```python
from build123d import *

# Parameters (mm, degrees)
SKETCH1_W           = 20
SKETCH1_H           = 50
BOSS_EXTRUDE1_DEPTH = 70
SKETCH2_R           = 2
SKETCH2_R_2         = 11.5
CUT_EXTRUDE2_DEPTH  = 60
SKETCH4_W           = 37
SKETCH4_H           = 15
CUT_EXTRUDE3_DEPTH  = 60
SKETCH8_R           = 2
CUT_EXTRUDE5_DEPTH  = 15
SKETCH9_W           = 42
SKETCH9_H           = 42
CUT_EXTRUDE6_DEPTH  = 6
CUT_EXTRUDE8_DEPTH  = 30
SKETCH12_W          = 20
SKETCH12_H          = 5
BOSS_EXTRUDE2_DEPTH = 10
BOSS_EXTRUDE3_DEPTH = 20
SKETCH15_R          = 2
CUT_EXTRUDE9_DEPTH  = 10
SKETCH17_R          = 3.5
CUT_EXTRUDE11_DEPTH = 8
SKETCH18_R          = 3.5
CUT_EXTRUDE12_DEPTH = 50


with BuildPart() as part:
    # Sketch1 → Boss-Extrude1 (new body)
    with BuildSketch(Plane(origin=(0, 0, 0), x_dir=(1, 0, 0), z_dir=(0, 1, 0))):
        with Locations((-10, -25)):
            Rectangle(SKETCH1_W, SKETCH1_H)
    extrude(amount=BOSS_EXTRUDE1_DEPTH)

    # Sketch2 → Cut-Extrude2 (cut)
    with BuildSketch(Plane(origin=(0, 0, 0), x_dir=(0, 0, -1), z_dir=(1, 0, 0))):
        with Locations((-9.5, 58)):
            Circle(SKETCH2_R)
        with Locations((-25, 42.5)):
            Circle(SKETCH2_R_2)
        with Locations((-9.5, 27)):
            Circle(SKETCH2_R)
        with Locations((-40.5, 27)):
            Circle(SKETCH2_R)
        with Locations((-40.5, 58)):
            Circle(SKETCH2_R)
    extrude(amount=-CUT_EXTRUDE2_DEPTH, mode=Mode.SUBTRACT)

    # Sketch4 → Cut-Extrude3 (cut)
    with BuildSketch(Plane(origin=(0, 0, 0), x_dir=(0, 0, -1), z_dir=(1, 0, 0))):
        with Locations((-31.5, 7.5)):
            Rectangle(SKETCH4_W, SKETCH4_H)
    extrude(amount=-CUT_EXTRUDE3_DEPTH, mode=Mode.SUBTRACT)

    # Sketch8 → Cut-Extrude5 (cut)
    with BuildSketch(Plane(origin=(0, 0, 0), x_dir=(-1, 0, 0), z_dir=(0, 0, -1))):
        with Locations((15, 6)):
            Circle(SKETCH8_R)
        with Locations((5, 6)):
            Circle(SKETCH8_R)
    extrude(amount=-CUT_EXTRUDE5_DEPTH, mode=Mode.SUBTRACT)

    # Sketch9 → Cut-Extrude6 (cut)
    with BuildSketch(Plane(origin=(0, 0, 0), x_dir=(0, 0, -1), z_dir=(1, 0, 0))):
        with Locations((-25, 42.5)):
            Rectangle(SKETCH9_W, SKETCH9_H)
    extrude(amount=-CUT_EXTRUDE6_DEPTH, mode=Mode.SUBTRACT)

    # Sketch11 → Cut-Extrude8 (cut)
    with BuildSketch(Plane(origin=(0, 0, 0), x_dir=(0, 0, -1), z_dir=(1, 0, 0))):
        Polygon((-7, 0), (0, 0), (0, 15), align=None)
    extrude(amount=-CUT_EXTRUDE8_DEPTH, mode=Mode.SUBTRACT)

    # Sketch12 → Boss-Extrude2 (add)
    with BuildSketch(Plane.XY.offset(50)):
        with Locations((-10, 17.5)):
            Rectangle(SKETCH12_W, SKETCH12_H)
    extrude(amount=BOSS_EXTRUDE2_DEPTH)

    # Sketch14 → Boss-Extrude3 (add)
    with BuildSketch(Plane(origin=(0, 0, 0), x_dir=(0, 0, -1), z_dir=(1, 0, 0))):
        Polygon((-50, 20), (-60, 20), (-50, 25), align=None)
    extrude(amount=-BOSS_EXTRUDE3_DEPTH)

    # Sketch15 → Cut-Extrude9 (cut)
    with BuildSketch(Plane(origin=(0, 15, 0), x_dir=(-1, 0, 0), z_dir=(0, -1, 0))):
        with Locations(Location((5, -55, 0), (0, 0, 90))):
            Circle(SKETCH15_R)
        with Locations(Location((15, -55, 0), (0, 0, 90))):
            Circle(SKETCH15_R)
    extrude(amount=-CUT_EXTRUDE9_DEPTH, mode=Mode.SUBTRACT)

    # Sketch17 → Cut-Extrude11 (cut)
    with BuildSketch(Plane(origin=(0, 0, 0), x_dir=(-1, 0, 0), z_dir=(0, 0, -1))):
        with Locations((15, 6)):
            Circle(SKETCH17_R)
        with Locations((5, 6)):
            Circle(SKETCH17_R)
    extrude(amount=-CUT_EXTRUDE11_DEPTH, mode=Mode.SUBTRACT)

    # Sketch18 → Cut-Extrude12 (cut)
    with BuildSketch(Plane(origin=(0, 70, 0), x_dir=(1, 0, 0), z_dir=(0, 1, 0))):
        with Locations(Location((-15, -55, 0), (0, 0, 270))):
            Circle(SKETCH18_R)
        with Locations(Location((-5, -55, 0), (0, 0, 270))):
            Circle(SKETCH18_R)
    extrude(amount=-CUT_EXTRUDE12_DEPTH, mode=Mode.SUBTRACT)


solid = part.part
```
Design review of the part built by this model. Coordinates are the model's own, in mm. A direction names the side the tool comes from. Round coordinates to 2 decimals unless told otherwise and drop trailing zeros. Write each loop counter-clockwise with the first axis right and the second up, starting at its lowest first coordinate (ties: lowest second). Pieces come first, ordered by that corner, then holes. Notation, with made-up numbers: (57.25, 71) -> (69.25, 71) arc R27 ccw to (69.25, 95) -> close; hole circle Ø6 at (6, -20). An arc over 180 degrees is marked (long way). Write item = value, one per line. Start each with the question number.
1) Tool access review of faces 4 (the face through (-10, 15, 36)), 5 (the face through (-3, 42, 4)), 6 (the face through (-17, 20, 57)), 7 (the face through (-4.54, 9.47, 5.83)): name each direction out of +Z, -Z, +X, -X, +Y, -Y from which nothing blocks a thin tool from reaching the whole face with its end or side.
2) Wall thickness on probe 1 along Y at (x, z) = (-2.75, 45); probe 2 along X at (y, z) = (20.95, 55); probe 3 along Y at (x, z) = (-12, 9.5): over which ranges is each line inside the solid? List them lowest first. Write a range as from..to.
3) Clearance check with flat-ended pins moving along their axes: pin 1 (2 mm diameter, centred on x = -3, z = 19, fed in from -Y); pin 2 (9 mm diameter, centred on x = -15, y = 6, fed in from -Z); pin 3 (3.5 mm diameter, centred on x = -5.5, y = 4.5, fed in from -Z); pin 4 (12 mm diameter, centred on y = 40, z = 26.5, fed in from +X). State where each tip first meets the part, or that it passes through.
4) Take a section at B-B, the plane y = 6. State the section outline as (x, z) points, plus the area to 3 significant figures.
5) Take a section at D-D, the plane x = -5. Count the separate pieces of the cut face and the enclosed holes in it, plus the area to 3 significant figures.
6) Take a section at C-C, the plane x = -9.75. State the section outline as (y, z) points.
7) Mouldability with a two-part tool opening along X and no side actions: class faces 1 (the face through (0, 20, 23)), 2 (the face through (-7, 20, 57)), 3 (the face through (-10, 70, 25)) as +X half, -X half, draft (parallel to the pull), parting line (faces both ways), or undercut.
8) Take a section at A-A, the plane z = 9.5. State the section outline as (x, y) points.
Results list:
q1.face_4 = +Z, +X, -X, -Y
q1.face_5 = +X
q1.face_6 = +Y
q1.face_7 = -Z
q2.probe_1 = 15..21.5, 63.5..70
q2.probe_2 = -20..-18.5, -11.5..-8.5, -1.5..0
q2.probe_3 = 0..25, 29..56, 60..70
q3.pin_1 = 15
q3.pin_2 = 2.1
q3.pin_3 = 8
q3.pin_4 = through
q4.outline = (-20, 4.2) -> (-18.5, 4.2) -> (-18.5, 8) -> (-17, 8) -> (-17, 13) -> (-20, 13) -> close; (-13, 8) -> (-11.5, 8) -> (-11.5, 4.2) -> (-8.5, 4.2) -> (-8.5, 8) -> (-7, 8) -> (-7, 13) -> (-13, 13) -> close; (-3, 8) -> (-1.5, 8) -> (-1.5, 4.2) -> (0, 4.2) -> (0, 13) -> (-3, 13) -> close
q4.area = 82.8 mm²
q5.separate_pieces = 3
q5.enclosed_holes = 1
q5.area = 1,120 mm²
q6.outline = (0, 7) -> (15, 0) -> (70, 0) -> (70, 50) -> (25, 50) -> (20, 60) -> (15, 60) -> (15, 13) -> (0, 13) -> close; hole circle Ø4 at (27, 9.5); hole circle Ø4 at (27, 40.5); hole circle Ø23 at (42.5, 25); hole circle Ø4 at (58, 9.5); hole circle Ø4 at (58, 40.5)
q7.face_1 = +X half
q7.face_2 = undercut
q7.face_3 = draft
q8.outline = (-20, 0) -> (0, 0) -> (0, 21.5) -> (-6, 21.5) -> (-6, 25) -> (-20, 25) -> close; (-20, 29) -> (-6, 29) -> (-6, 56) -> (-20, 56) -> close; (-20, 60) -> (-6, 60) -> (-6, 63.5) -> (0, 63.5) -> (0, 70) -> (-20, 70) -> close; hole circle Ø4 at (-15, 6); hole circle Ø4 at (-5, 6)
